Build history of the part. All positions in model axes, mm. A direction names the side the tool comes from. Round coordinates to 2 decimals unless told otherwise and drop trailing zeros. Loops run counter-clockwise (first coordinate to the right, second up) from the corner with the lowest first, then second, coordinate; pieces in that order, holes last. Notation, with made-up numbers: M 26.5,42 L 52.5,42 A17 cw 52.5,51 Z; hole C 57.5,86 d11. An arc over 180 degrees is marked long. One line per item, written item: value.
```python
from build123d import *

# Parameters (mm, degrees)
SKETCH1_R           = 9.25
BOSS_EXTRUDE1_DEPTH = 12
SKETCH2_R           = 5.95
CUT_EXTRUDE1_DEPTH  = 4
CUT_EXTRUDE2_DEPTH  = 3
CIRPATTERN1_COUNT   = 8
SKETCH5_R           = 3.175
CUT_EXTRUDE3_DEPTH  = 8
CUT_EXTRUDE4_START  = -5
SKETCH6_R           = 5.95
CUT_EXTRUDE4_DEPTH  = 2
CUT_EXTRUDE5_REACH  = 19.752
SKETCH7_R           = 5.675
SKETCH8_R           = 1.5
FILLET1_R           = 1


with BuildPart() as part:
    # Sketch1 → Boss-Extrude1 (new body)
    with BuildSketch(Plane.XY):
        Circle(SKETCH1_R)
    extrude(amount=BOSS_EXTRUDE1_DEPTH)

    # Sketch2 → Cut-Extrude1 (cut)
    with BuildSketch(Plane(origin=(0, 0, 0), x_dir=(-1, 0, 0), z_dir=(0, 0, -1))):
        Circle(SKETCH2_R)
    extrude(amount=-CUT_EXTRUDE1_DEPTH, mode=Mode.SUBTRACT)

    # Sketch4 → Cut-Extrude2 (cut)
    with BuildSketch(Plane(origin=(0, 0, 0), x_dir=(-1, 0, 0), z_dir=(0, 0, -1))):
        with BuildLine():
            Line((1, 5.865364439), (1, 8.865364439))
            Line((1, 8.865364439), (-1, 8.865364439))
            Line((-1, 8.865364439), (-1, 5.865364439))
            ThreePointArc((-1, 5.865364439), (0, 5.95), (1, 5.865364439))
        make_face()
    cut_extrude2 = extrude(amount=-CUT_EXTRUDE2_DEPTH, mode=Mode.SUBTRACT)

    # CirPattern1: Cut-Extrude2 ×8 about axis
    cirpattern1_axis = Axis((0, 0, 0), (0, 0, 1))
    for i in range(1, CIRPATTERN1_COUNT):
        add(cut_extrude2.rotate(cirpattern1_axis, i * 360 / CIRPATTERN1_COUNT), mode=Mode.SUBTRACT)

    # Sketch5 → Cut-Extrude3 (cut)
    with BuildSketch(Plane.XY.offset(12)):
        Circle(SKETCH5_R)
    extrude(amount=-CUT_EXTRUDE3_DEPTH, mode=Mode.SUBTRACT)

    # Sketch6 → Cut-Extrude4 (cut)
    with BuildSketch(Plane.XY.offset(12).offset(CUT_EXTRUDE4_START)):
        with Locations(Location((0, 0, 0), (0, 0, 180))):
            Circle(SKETCH6_R)
    extrude(amount=CUT_EXTRUDE4_DEPTH, mode=Mode.SUBTRACT)

    # Sketch7 → Cut-Extrude5 (cut, up to next)
    with BuildSketch(Plane.XY.offset(12), mode=Mode.PRIVATE) as cut_extrude5_sk1:
        Circle(SKETCH7_R)
    cut_extrude5_tool1 = extrude(cut_extrude5_sk1.sketch, amount=-CUT_EXTRUDE5_REACH, mode=Mode.PRIVATE) & part.part
    add(cut_extrude5_tool1.solids().sort_by_distance((0, 0, 12))[0], mode=Mode.SUBTRACT)

    # Sketch8 → Cut-Revolve1 (revolve, cut)
    with BuildSketch(Plane(origin=(0, 0, 0), x_dir=(1, 0, 0), z_dir=(0, 1, 0)), mode=Mode.PRIVATE) as cut_revolve1_sk:
        with Locations((-4.43, -10.5)):
            Circle(SKETCH8_R)
    revolve(cut_revolve1_sk.sketch.rotate(Axis((0, 0, 0), (0, 0, 1)), 180), axis=Axis((0, 0, 0), (0, 0, 1)), mode=Mode.SUBTRACT)

    # Fillet1
    fillet1_edges = [part.edges().sort_by_distance(p)[0] for p in [
        (-1, 5.865364439, 1.5),
        (1, 5.865364439, 1.5),
        (-5.865364439, -1, 1.5),
        (-5.865364439, 1, 1.5),
        (-3.440332188, -4.85454575, 1.5),
        (-4.85454575, -3.440332188, 1.5),
        (1, -5.865364439, 1.5),
        (-1, -5.865364439, 1.5),
        (4.85454575, -3.440332188, 1.5),
        (3.440332188, -4.85454575, 1.5),
        (5.865364439, 1, 1.5),
        (5.865364439, -1, 1.5),
        (3.440332188, 4.85454575, 1.5),
        (4.85454575, 3.440332188, 1.5),
        (-4.85454575, 3.440332188, 1.5),
        (-3.440332188, 4.85454575, 1.5),
    ]]
    fillet(fillet1_edges, radius=FILLET1_R)


solid = part.part
```
Item 1: Slice it at C-C, the plane z = 3.5. Give the cut face in (x, y).
Check values:
outline: C 0,0 d18.5; hole C 0,0 d11.9
Item 2: Drop flat-ended pins along their axis: P1, Ø0.7, axis at y = -8, z = 2, coming from the +X side; P2, Ø3.5, axis at x = 0.5, y = 1.5, coming from the -Z side; P3, Ø2, axis at x = -2.5, z = 1.5, coming from the -Y side. Give the stop position or say it passes through.
Check values:
P1: stops at x = 5.2
P2: stops at z = 4
P3: stops at y = -9.13
Item 3: Slice it at A-A, the plane y = 0. Give the cut face in (x, z) (3 decimals), and give its area (3 significant figures).
Check values:
outline: M -9.25,0 L -8.865,0 L -8.865,3 L -5.95,3 L -5.95,4 L -3.175,4 L -3.175,7 L -5.95,7 L -5.95,9 L -5.675,9 L -5.675,9.663 A1.5 cw -5.675,11.337 L -5.675,12 L -9.25,12 Z; M 3.175,4 L 5.95,4 L 5.95,3 L 8.865,3 L 8.865,0 L 9.25,0 L 9.25,12 L 5.675,12 L 5.675,11.337 A1.5 cw 5.675,9.663 L 5.675,9 L 5.95,9 L 5.95,7 L 3.175,7 Z
area: 79.4 mm2
Item 4: Which spindle directions (+Z, -Z, +X, -X, +Y, -Y) get a long thin tool onto all of the face, cutting with end or side? Do faces 1 (the face through (0, -6, 12)), 2 (the face through (-6.052, -1.203, 1.521)). Say none if no direction does.
Check values:
face 1: +Z, +X, -X, +Y, -Y
face 2: -Z
Item 5: Slice it at D-D, the plane x = -7.75. Give the cut face in (y, z).
Check values:
outline: M -5.05,0 L -1,0 L -1,3 L 1,3 L 1,0 L 5.05,0 L 5.05,12 L -5.05,12 Z
Item 6: Wall check: line 1 along Y through (x, z) = (0, 7.9); line 2 along Y through (x, z) = (0, 1.35); line 3 along X through (y, z) = (-5.25, 1.25). Give the ranges that are in metal, low to high.
Check values:
line 1: y = -9.25 to -5.95, 5.95 to 9.25
line 2: y = -9.25 to -8.87, 8.87 to 9.25
line 3: x = -7.62 to -6.66, -3.78 to -2.8, 2.8 to 3.78, 6.66 to 7.62
